Verification items for the finished model (mm, model axes). Face numbers are marked on the shaded views. A direction names the side the tool comes from. Round coordinates to 2 decimals unless told otherwise and drop trailing zeros. Order: outer loops, then holes, each group sorted by start corner. A loop starts at its lowest first (then second) coordinate and runs counter-clockwise, first axis right, second up. Notation, with made-up numbers: (15.25, 73.5) -> (57.25, 73.5) arc R5 ccw to (57.25, 80.5) -> close; hole circle Ø5 at (58.25, 11.25). An arc over 180 degrees is marked (long way). Put each result on its own line as item: value.
```python
from build123d import *

# Parameters (mm, degrees)
SKETCH1_W           = 139.5
SKETCH1_H           = 126
BOSS_EXTRUDE1_DEPTH = 27
SKETCH2_W           = 115.5
SKETCH2_H           = 102
CUT_EXTRUDE1_DEPTH  = 7
SKETCH3_W           = 115.5
SKETCH3_H           = 85
CUT_EXTRUDE2_DEPTH  = 7
SKETCH4_W           = 12
SKETCH4_H           = 66
CUT_EXTRUDE3_DEPTH  = 14
SKETCH5_W           = 12
SKETCH5_H           = 66
CUT_EXTRUDE4_DEPTH  = 14
CUT_EXTRUDE5_DEPTH  = 7
FILLET1_R           = 2.5


with BuildPart() as part:
    # Sketch1 → Boss-Extrude1 (new body)
    with BuildSketch(Plane(origin=(0, 0, 0), x_dir=(1, 0, 0), z_dir=(0, 1, 0))):
        with Locations((69.75, 63)):
            Rectangle(SKETCH1_W, SKETCH1_H)
    extrude(amount=BOSS_EXTRUDE1_DEPTH)

    # Sketch2 → Cut-Extrude1 (cut)
    with BuildSketch(Plane(origin=(0, 27, 0), x_dir=(1, 0, 0), z_dir=(0, 1, 0))):
        with Locations((69.75, 63)):
            Rectangle(SKETCH2_W, SKETCH2_H)
    extrude(amount=-CUT_EXTRUDE1_DEPTH, mode=Mode.SUBTRACT)

    # Sketch3 → Cut-Extrude2 (cut)
    with BuildSketch(Plane(origin=(0, 20, 0), x_dir=(1, 0, 0), z_dir=(0, 1, 0))):
        with Locations((69.75, 63)):
            Rectangle(SKETCH3_W, SKETCH3_H)
    extrude(amount=-CUT_EXTRUDE2_DEPTH, mode=Mode.SUBTRACT)

    # Sketch4 → Cut-Extrude3 (cut)
    with BuildSketch(Plane(origin=(0, 27, 0), x_dir=(1, 0, 0), z_dir=(0, 1, 0))):
        with Locations((6, 63)):
            Rectangle(SKETCH4_W, SKETCH4_H)
    extrude(amount=-CUT_EXTRUDE3_DEPTH, mode=Mode.SUBTRACT)

    # Sketch5 → Cut-Extrude4 (cut)
    with BuildSketch(Plane(origin=(0, 27, 0), x_dir=(1, 0, 0), z_dir=(0, 1, 0))):
        with Locations((133.5, 63)):
            Rectangle(SKETCH5_W, SKETCH5_H)
    extrude(amount=-CUT_EXTRUDE4_DEPTH, mode=Mode.SUBTRACT)

    # Sketch6 → Cut-Extrude5 (cut)
    with BuildSketch(Plane(origin=(0, 27, 0), x_dir=(1, 0, 0), z_dir=(0, 1, 0))):
        with BuildLine():
            Line((12, 12), (17, 12))
            ThreePointArc((17, 12), (14.5, 9.5), (12, 12))
        make_face()
        with BuildLine():
            Line((122.5, 12), (127.5, 12))
            ThreePointArc((127.5, 12), (125, 9.5), (122.5, 12))
        make_face()
        with BuildLine():
            Line((12, 114), (17, 114))
            ThreePointArc((17, 114), (14.5, 116.5), (12, 114))
        make_face()
        with BuildLine():
            Line((122.5, 114), (127.5, 114))
            ThreePointArc((127.5, 114), (125, 116.5), (122.5, 114))
        make_face()
    extrude(amount=-CUT_EXTRUDE5_DEPTH, mode=Mode.SUBTRACT)

    # Fillet1
    fillet1_edges = [part.edges().sort_by_distance(p)[0] for p in [
        (127.5, 16.5, -105.5),
        (127.5, 16.5, -20.5),
        (12, 16.5, -20.5),
        (12, 16.5, -105.5),
    ]]
    fillet(fillet1_edges, radius=FILLET1_R)


solid = part.part
```
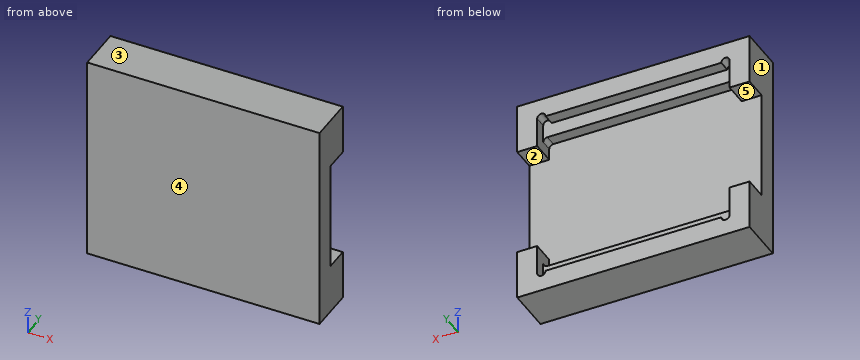
Item 1: Sectioned sample at C-C, the plane z = -59. Record the boundary of the cut face in (x, y).
Geometry check:
outline: (0, 0) -> (139.5, 0) -> (139.5, 13) -> (0, 13) -> close
Item 2: Release check for a two-part mould opening along Z. For the marked faces 1, 2 and 3 record: pulls with the +Z half, pulls with the -Z half, needs draft (parallel to the pull), parting line crosses it, or undercut.
Geometry check:
face 1: needs draft
face 2: undercut
face 3: pulls with the +Z half
Item 3: Sectioned sample at B-B, the plane x = 67. Record the boundary of the cut face in (y, z), then the cut area to 3 significant figures.
Geometry check:
outline: (0, -126) -> (27, -126) -> (27, -114) -> (20, -114) -> (20, -105.5) -> (13, -105.5) -> (13, -20.5) -> (20, -20.5) -> (20, -12) -> (27, -12) -> (27, 0) -> (0, 0) -> close
area: 2,090 mm2
Item 4: Sectioned sample at A-A, the plane y = 21.75. Record the boundary of the cut face in (x, z), then the cut area to 3 significant figures.
Geometry check:
outline: (0, -126) -> (139.5, -126) -> (139.5, -96) -> (127.5, -96) -> (127.5, -114) arc R2.5 cw to (122.5, -114) -> (17, -114) arc R2.5 cw to (12, -114) -> (12, -96) -> (0, -96) -> close; (0, -30) -> (12, -30) -> (12, -12) arc R2.5 cw to (17, -12) -> (122.5, -12) arc R2.5 cw to (127.5, -12) -> (127.5, -30) -> (139.5, -30) -> (139.5, 0) -> (0, 0) -> close
area: 4,170 mm2
Item 5: Material ranges on line 1 along Z through (x, y) = (74.5, 22.75); line 2 along Z through (x, y) = (103, 19.5); line 3 along Y through (x, z) = (23, -85), recorded low to high.
Geometry check:
line 1: -126 to -114, -12 to 0
line 2: -126 to -105.5, -20.5 to 0
line 3: 0 to 13
Item 6: Tool access check on the marked faces 4 and 5. Record the directions out of +Z, -Z, +X, -X, +Y, -Y that give a thin tool (end or side, any length) a straight path to the whole face; none if there is none.
Geometry check:
face 4: +Z, -Z, +X, -X, -Y
face 5: +X, -X, +Y
Item 7: Depth check by flat-ended pin: pin 1 Ø15.5 at (y, z) = (22.5, -18.5) entering from -X; pin 2 Ø5 at (x, z) = (29, -42.5) entering from +Y. Enter the tip coordinate at first touch or a pass-through.
Geometry check:
pin 1: x = 0
pin 2: y = 13
